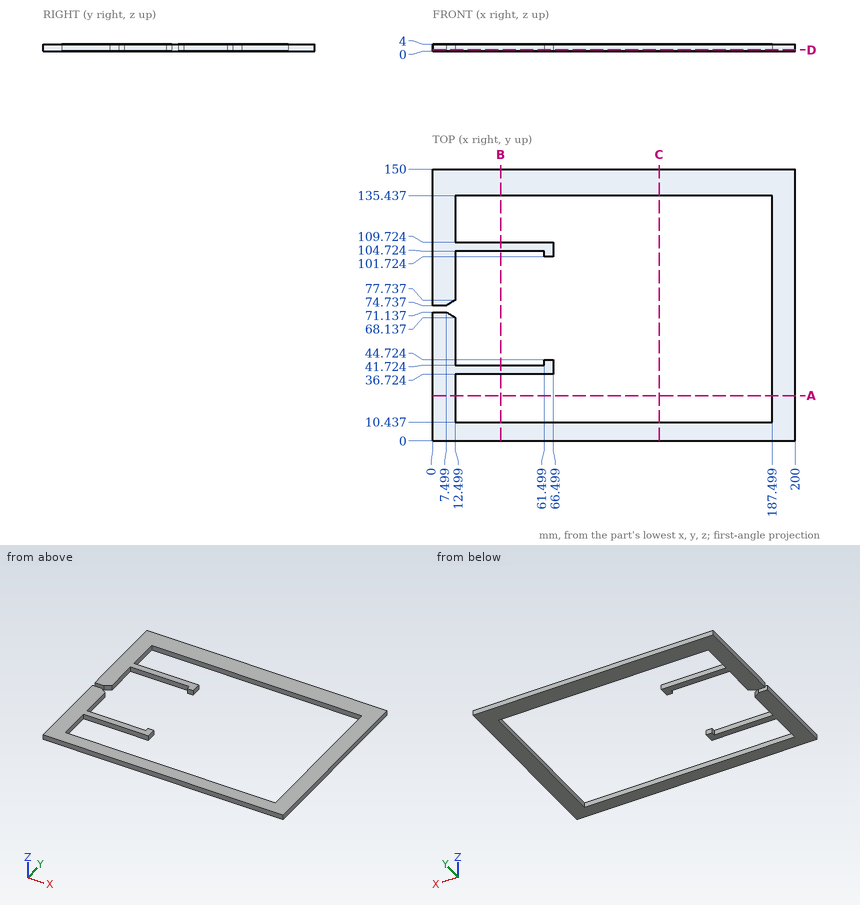
Design review of the part shown in the three views and the two pictorial views. Dimensions are in mm from the part's minimum x, y and z. Round coordinates to 2 decimals unless told otherwise and drop trailing zeros. Loops run counter-clockwise (first coordinate to the right, second up) from the corner with the lowest first, then second, coordinate; pieces in that order, holes last.
Q1. Add section A-A on y = 25. Write out the cut boundary in (x, z).
Result sheet:
outline: (0, 0) - (12.5, 0) - (12.5, 4) - (0, 4) - close; (187.5, 0) - (200, 0) - (200, 4) - (187.5, 4) - close
Q2. Add section B-B on x = 37.5. Write out the cut boundary in (y, z), plus the area to 3 significant figures.
Result sheet:
outline: (0, 0) - (10.44, 0) - (10.44, 4) - (0, 4) - close; (36.72, 0) - (41.72, 0) - (41.72, 4) - (36.72, 4) - close; (104.72, 0) - (109.72, 0) - (109.72, 4) - (104.72, 4) - close; (135.44, 0) - (150, 0) - (150, 4) - (135.44, 4) - close
area: 140 mm2
Q3. To check wall thickness, follow line 1 along Y through (x, z) = (56.5, 1.25); line 2 along X through (y, z) = (63, 1.9); line 3 along Y through (x, z) = (95, 2). State the ranges of each line that lie inside material, in increasing order.
Result sheet:
line 1: y = 0 to 10.44, 36.72 to 41.72, 104.72 to 109.72, 135.44 to 150
line 2: x = 0 to 12.5, 187.5 to 200
line 3: y = 0 to 10.44, 135.44 to 150
Q4. Add section D-D on z = 0.8. Write out the cut boundary in (x, y).
Result sheet:
outline: (0, 0) - (200, 0) - (200, 150) - (0, 150) - (0, 74.74) - (7.5, 74.74) - (12.5, 77.74) - (12.5, 104.72) - (61.5, 104.72) - (61.5, 101.72) - (66.5, 101.72) - (66.5, 109.72) - (12.5, 109.72) - (12.5, 135.44) - (187.5, 135.44) - (187.5, 10.44) - (12.5, 10.44) - (12.5, 36.72) - (66.5, 36.72) - (66.5, 44.72) - (61.5, 44.72) - (61.5, 41.72) - (12.5, 41.72) - (12.5, 68.14) - (7.5, 71.14) - (0, 71.14) - close
Q5. Add section C-C on x = 125. Write out the cut boundary in (y, z), plus the area to 3 significant figures.
Result sheet:
outline: (0, 0) - (10.44, 0) - (10.44, 4) - (0, 4) - close; (135.44, 0) - (150, 0) - (150, 4) - (135.44, 4) - close
area: 100 mm2
